Build history of the part. All positions in model axes, mm. A direction names the side the tool comes from. Round coordinates to 2 decimals unless told otherwise and drop trailing zeros. Order: outer loops, then holes, each group sorted by start corner. A loop starts at its lowest first (then second) coordinate and runs counter-clockwise, first axis right, second up. Notation, with made-up numbers: M -19.75,41 L 34.25,41 A16 ccw 34.25,72 Z; hole C -21,1.25 d11. An arc over 180 degrees is marked long. One line per question, with ' | ' between items. Start each with the question number.
from build123d import *

# Parameters (mm, degrees)
SKETCH1_W               = 140
SKETCH1_H               = 88
BOSS_EXTRUDE1_DEPTH     = 16
FILLET1_R               = 15
HOLE2_D                 = 9
HOLE2_CBORE_D           = 15
HOLE2_CBORE_DEPTH       = 5
SWEEP1_PROFILE_R        = 22.5
CUT_SWEEP1_PROFILE_R    = 6
BOSS_EXTRUDE2_START     = 50
SKETCH21_R              = 28
BOSS_EXTRUDE2_DEPTH     = 40
BOSS_EXTRUDE3_DEPTH     = 10
CUT_EXTRUDE1_DEPTH      = 6
SKETCH27_R              = 12
BOSS_EXTRUDE4_DEPTH     = 16
CUT_EXTRUDE2_REACH      = 155.379
SKETCH28_R              = 7
CUT_SWEEP2_PROFILE_R    = 6
BOSS_EXTRUDE5_START     = -5
BOSS_EXTRUDE5_DEPTH     = 15
CUT_SWEEP3_PROFILE_R    = 15
SKETCH57_R              = 17.5
CUT_EXTRUDE3_DEPTH      = 56.4
CUT_EXTRUDE4_DEPTH      = 224.949486459
CUT_EXTRUDE4_DEPTH_BACK = 224.949486459


with BuildPart() as part:
    # Sketch1 → Boss-Extrude1 (new body)
    with BuildSketch(Plane(origin=(0, 0, 0), x_dir=(1, 0, 0), z_dir=(0, 1, 0))):
        Rectangle(SKETCH1_W, SKETCH1_H)
    extrude(amount=BOSS_EXTRUDE1_DEPTH)

    # Fillet1
    fillet1_edges = [part.edges().sort_by_distance(p)[0] for p in [
        (70, 8, 44),
        (-70, 8, 44),
        (-70, 8, -44),
        (70, 8, -44),
    ]]
    fillet(fillet1_edges, radius=FILLET1_R)

    # Hole2 (through all)
    with Locations(Plane(origin=(0, 16, 0), x_dir=(1, 0, 0), z_dir=(0, 1, 0))):
        with Locations((-55, 29), (55, 29), (-55, -29), (55, -29)):
            CounterBoreHole(HOLE2_D / 2, HOLE2_CBORE_D / 2, HOLE2_CBORE_DEPTH)

    # Sweep1: sweep along a path in Sketch6
    with BuildLine(Plane(origin=(0, 0, 0), x_dir=(0, 0, -1), z_dir=(1, 0, 0))) as sweep1_path:
        Line((0, 0), (0, 105.475997542))
        ThreePointArc((0, 105.475997542), (2.860918449, 118.701500419), (10.932120397, 129.562185473))
        Line((10.932120397, 129.562185473), (54.193922845, 167.402729106))
    # Sweep1 profile (on start of the path) → Sweep1 (sweep)
    with BuildSketch(Plane.ZX):
        Circle(SWEEP1_PROFILE_R)
    sweep(path=sweep1_path.line)

    # Cut-Sweep1: sweep along a path in Sketch6_5
    with BuildLine(Plane(origin=(0, 0, 0), x_dir=(0, 0, -1), z_dir=(1, 0, 0))) as cut_sweep1_path:
        Line((0, 0), (0, 105.475997542))
        ThreePointArc((0, 105.475997542), (2.860918449, 118.701500419), (10.932120397, 129.562185473))
        Line((10.932120397, 129.562185473), (54.193922845, 167.402729106))
    # Cut-Sweep1 profile (on start of the path) → Cut-Sweep1 (sweep, cut)
    with BuildSketch(Plane.ZX):
        Circle(CUT_SWEEP1_PROFILE_R)
    sweep(path=cut_sweep1_path.line, mode=Mode.SUBTRACT)

    # Sketch21 → Boss-Extrude2 (add)
    with BuildSketch(Plane(origin=(0, 0, 0), x_dir=(1, 0, 0), z_dir=(0, 1, 0)).offset(BOSS_EXTRUDE2_START)):
        with Locations(Location((0, 0, 0), (0, 0, 270))):
            Circle(SKETCH21_R)
    extrude(amount=BOSS_EXTRUDE2_DEPTH)

    # Sketch23 → Boss-Extrude3 (add, symmetric)
    with BuildSketch(Plane(origin=(0, 70, 0), x_dir=(1, 0, 0), z_dir=(0, 1, 0))):
        with BuildLine():
            Line((-27.6458869, -4.43902439), (-14.810296553, -84.37804878))
            ThreePointArc((-14.810296553, -84.37804878), (0, -97), (14.810296553, -84.37804878))
            Line((14.810296553, -84.37804878), (27.6458869, -4.43902439))
            ThreePointArc((27.6458869, -4.43902439), (0, 28), (-27.6458869, -4.43902439))
        make_face()
    extrude(amount=BOSS_EXTRUDE3_DEPTH, both=True)

    # Sketch25 → Cut-Extrude1 (cut, symmetric)
    with BuildSketch(Plane(origin=(0, 70, 0), x_dir=(1, 0, 0), z_dir=(0, 1, 0))):
        with BuildLine():
            Line((10.860884139, -83.743902439), (23.696474485, -3.804878049))
            ThreePointArc((23.696474485, -3.804878049), (0, 24), (-23.696474485, -3.804878049))
            Line((-23.696474485, -3.804878049), (-10.860884139, -83.743902439))
            ThreePointArc((-10.860884139, -83.743902439), (0, -93), (10.860884139, -83.743902439))
        make_face()
    extrude(amount=CUT_EXTRUDE1_DEPTH, both=True, mode=Mode.SUBTRACT)

    # Sketch27 → Boss-Extrude4 (add)
    with BuildSketch(Plane(origin=(0, 80, 0), x_dir=(1, 0, 0), z_dir=(0, 1, 0))):
        with Locations(Location((0, -82, 0), (0, 0, 270))):
            Circle(SKETCH27_R)
    extrude(amount=BOSS_EXTRUDE4_DEPTH)

    # Sketch28 → Cut-Extrude2 (cut, up to next)
    with BuildSketch(Plane(origin=(0, 96, 0), x_dir=(1, 0, 0), z_dir=(0, 1, 0)), mode=Mode.PRIVATE) as cut_extrude2_sk1:
        with Locations(Location((0, -82, 0), (0, 0, 270))):
            Circle(SKETCH28_R)
    cut_extrude2_tool1 = extrude(cut_extrude2_sk1.sketch, amount=-CUT_EXTRUDE2_REACH, mode=Mode.PRIVATE) & part.part
    add(cut_extrude2_tool1.solids().sort_by_distance((0, 96, 82))[0], mode=Mode.SUBTRACT)

    # Sketch30 → Cut-Revolve1 (revolve, cut)
    with BuildSketch(Plane(origin=(0, 0, 0), x_dir=(0, 0, -1), z_dir=(1, 0, 0)), mode=Mode.PRIVATE) as cut_revolve1_sk:
        Polygon((0, 0), (18.5, 0), (18.5, 54), (24, 54), (24, 86), (0, 86), align=None)
    revolve(cut_revolve1_sk.sketch.rotate(Axis((0, 86, 0), (0, -1, 0)), 180), axis=Axis((0, 86, 0), (0, -1, 0)), mode=Mode.SUBTRACT)

    # Cut-Sweep2: sweep along a path in Sketch6_6
    with BuildLine(Plane(origin=(0, 0, 0), x_dir=(0, 0, -1), z_dir=(1, 0, 0))) as cut_sweep2_path:
        Line((0, 0), (0, 105.475997542))
        ThreePointArc((0, 105.475997542), (2.860918449, 118.701500419), (10.932120397, 129.562185473))
        Line((10.932120397, 129.562185473), (54.193922845, 167.402729106))
    # Cut-Sweep2 profile (on start of the path) → Cut-Sweep2 (sweep, cut)
    with BuildSketch(Plane.ZX):
        Circle(CUT_SWEEP2_PROFILE_R)
    sweep(path=cut_sweep2_path.line, mode=Mode.SUBTRACT)

    # Sketch41 → Boss-Extrude5 (add)
    with BuildSketch(Plane(origin=(0, 99.417051483, -113.660122933), x_dir=(-1, 0, 0), z_dir=(0, 0.6583712375823932, -0.752693372844632)).offset(BOSS_EXTRUDE5_START)):
        Polygon((19.341234018, 56.823204741), (38.682468036, 90.323204741), (19.341234018, 123.823204741), (-19.341234018, 123.823204741), (-38.682468036, 90.323204741), (-19.341234018, 56.823204741), align=None)
    extrude(amount=-BOSS_EXTRUDE5_DEPTH)

    # Cut-Sweep3: sweep along a path in Sketch43
    with BuildLine(Plane(origin=(0, 0, 0), x_dir=(0, 0, -1), z_dir=(1, 0, 0))) as cut_sweep3_path:
        Line((54.193922845, 167.402729106), (10.932120397, 129.562185473))
        ThreePointArc((10.932120397, 129.562185473), (6.509742227, 124.821455889), (3.133658129, 119.286656721))
    # Cut-Sweep3 profile (on start of the path) → Cut-Sweep3 (sweep, cut)
    with BuildSketch(Plane(origin=(0, 167.402729106, -54.193922845), x_dir=(0, 0.7526933728446314, 0.6583712375823938), z_dir=(0, -0.6583712375823938, 0.7526933728446314))):
        Circle(CUT_SWEEP3_PROFILE_R)
    sweep(path=cut_sweep3_path.line, mode=Mode.SUBTRACT)

    # Sketch57 → Cut-Extrude3 (cut)
    with BuildSketch(Plane(origin=(0, 99.417051483, -113.660122933), x_dir=(-1, 0, 0), z_dir=(0, 0.6583712375823932, -0.752693372844632))):
        with Locations(Location((0, 90.323204741, 0), (0, 0, 90))):
            Circle(SKETCH57_R)
    extrude(amount=-CUT_EXTRUDE3_DEPTH, mode=Mode.SUBTRACT)

    # Sketch59 → Cut-Extrude4 (cut, two sides: drawn at the far end of the back side and taken through both)
    with BuildSketch(Plane.XY.offset(-CUT_EXTRUDE4_DEPTH_BACK)):
        Polygon((-35, 0), (35, 0), (32, 3), (-32, 3), align=None)
    extrude(amount=CUT_EXTRUDE4_DEPTH + CUT_EXTRUDE4_DEPTH_BACK, mode=Mode.SUBTRACT)


solid = part.part
Item 1: Cut at A-A on y = 92.5. Write the cut outline in (x, z), then the cut area to 3 significant figures.
Item 2: Two-plate mould, pull along X, no slides. Class faces 4 (the face through (13.04, 124.35, -16.92)), 5 (the face through (29.147, 146.811, -55.738)), 6 (the face through (0, 70, 97)): +X half, -X half, draft (parallel to the pull), parting line (faces both ways), or undercut.
Item 3: Cut at B-B on x = 0. Count the separate pieces of the cut face and the enclosed holes in it, then the cut area to 3 significant figures.
Item 4: Wall check: line 1 along Z through (x, y) = (-55, 14); line 2 along Y through (x, z) = (-5.5, 66); line 3 along Y through (x, z) = (17.5, 24). Give the ranges that are in metal, low to high. Write a range as [from, to].
Item 5: Tool access for faces 1 (the face through (1.231, 69.72, -27.973)), 2 (the face through (-5.2, 96, 87.2)), 3 (the face through (-1, 8, 44)): list every direction of +Z, -Z, +X, -X, +Y, -Y with a clear straight run to the whole face (end or side of a thin tool).
Item 6: Flat gauge pins, fed straight in: pin 1 (1.5 mm diameter, centred on y = 66.5, z = -9, fed in from +X); pin 2 (8 mm diameter, centred on x = 55, z = -29, fed in from +Y); pin 3 (7 mm diameter, centred on x = 0.5, z = 84.5, fed in from +Y); pin 4 (6 mm diameter, centred on x = -33, z = 7, fed in from +Y). Where does each tip first touch, or does it go through?
Results found:
1) outline: C 0,0 d45; C 0,82 d24; hole C 0,82 d14; hole C 0,0 d12 | area: 1,780 mm^2
2) face 4: undercut | face 5: +X half | face 6: parting line
3) separate pieces: 3 | enclosed holes: 0 | area: 4,190 mm^2
4) line 1: z = [-44, -36.5], [-21.5, 21.5], [36.5, 44] | line 2: y = [60, 64], [76, 80] | line 3: y = [3, 16], [60, 64], [76, 80]
5) face 1: none | face 2: +Z, +X, -X, +Y | face 3: +Z, +X, -X, -Y
6) pin 1: stops at x = 26.76 | pin 2: passes through | pin 3: stops at y = 64 | pin 4: stops at y = 16
